Autodesk Inventor part; units mm, degrees
ref_plane "YZ Plane" through (0, 0, 0) normal (1, 0, 0) x (0, 1, 0)
ref_plane "XZ Plane" through (0, 0, 0) normal (0, 1, 0) x (-1, 0, 0)
ref_plane "XY Plane" through (0, 0, 0) normal (0, 0, 1) x (1, 0, 0)
sketch "Sketch1" plane through (0, 0, 0) normal (0, 0, 1) x (1, 0, 0)
  line L0 (-32.5, 16.5) -> (32.5, 16.5)
  line L1 (32.5, 16.5) -> (32.5, -16.5)
  line L2 (32.5, -16.5) -> (-32.5, -16.5)
  line L3 (-32.5, -16.5) -> (-32.5, 16.5)
  line L4 (-32.5, 16.5) -> (32.5, -16.5) construction
  line L5 (32.5, 16.5) -> (-32.5, -16.5) construction
  point P0 (0, 0)
  dimension "d0" = 65
  dimension "d1" = 33
extrude "Extrusion1" add sketch "Sketch1" along normal blind 66
shell "Shell1" thickness 3 removed faces 1 at (-10.8333, 5.5, 66)
sketch "Sketch2" plane through (-32.5, -16.5, 0) normal (0, -1, 0) x (1, 0, 0)
  line L0 (33.5, 65) -> (31.5, 65)
  line L1 (27.5, 61) -> (27.5, 9)
  line L2 (31.5, 5) -> (33.5, 5)
  line L3 (37.5, 9) -> (37.5, 61)
  line L4 (32.5, 0) -> (32.5, 66) construction
  line L5 (65, 66) -> (0, 66)
  line L6 (0, 0) -> (65, 0)
  arc A0 (33.5, 5) -> (37.5, 9) centre (33.5, 9) ccw
  arc A1 (27.5, 9) -> (31.5, 5) centre (31.5, 9) ccw
  arc A2 (37.5, 61) -> (33.5, 65) centre (33.5, 61) ccw
  arc A3 (31.5, 65) -> (27.5, 61) centre (31.5, 61) ccw
  point P0 (37.5, 65)
  point P1 (27.5, 65)
  point P2 (27.5, 5)
  point P3 (37.5, 5)
  dimension "d5" = 10
  dimension "d6" = 60
  dimension "d7" = 5
  dimension "d10" = 4
extrude "Extrusion2" cut sketch "Sketch2" against normal up to surface (30 mm away)
sketch "Sketch3" plane through (0, 0, 0) normal (0, 0, -1) x (-1, 0, 0)
  line L0 (32.5, 16.5) -> (32.5, -16.5)
  line L1 (32.5, 0) -> (-32.5, 0) construction
  line L2 (-32.5, -16.5) -> (-32.5, 16.5)
  circle A0 centre (-15, -8) radius 2.5
  circle A1 centre (-15, 8) radius 2.5
  circle A2 centre (15, -8) radius 2.5
  circle A3 centre (15, 8) radius 2.5
  point P0 (0, 0)
  point P1 (0, 0)
  dimension "d11" = 5
  dimension "d12" = 5
  dimension "d13" = 5
  dimension "d14" = 5
  dimension "d15" = 8
  dimension "d16" = 8
  dimension "d17" = 30
  dimension "d18" = 15
extrude "Extrusion3" cut sketch "Sketch3" against normal through all
properties part number "SLIDER" material "Steel, Alloy"
Input: part model. Units: mm. Frame: model coordinates. A direction names the side the tool comes from. Give positions to 0.01 mm unless a question says otherwise; leave off trailing zeros. Order: outer loops, then holes, each group sorted by start corner. A loop starts at its lowest first (then second) coordinate and runs counter-clockwise, first axis right, second up. Notation, with made-up numbers: (16.25, -23.5) -> (68.25, -23.5) arc R27 ccw to (68.25, -1.5) -> close; hole circle Ø1 at (-33.75, 12). An arc over 180 degrees is marked (long way). Write each question's results on one line, items separated by ' | '. Start each with the question number.
Item 1: Contact query for a flat-ended pin moving along its axis: P1, Ø8, axis at x = 5.5, y = -2, coming from the +Z side. Output: stop coordinate, or through.
Item 2: Line query: line 1 (Y direction, x = -15, z = 1); line 2 (X direction, y = 5.5, z = 53); line 3 (Y direction, x = 21.5, z = 33.5). Output: solid intervals per line, ascending.
Item 3: Set-up query: faces 4 (the flat face through (8, -16.5, 33)), 5 (the flat face through (29.5, 0, 34)), 6 (the flat face through (0, -15, 65)). Return all of +Z, -Z, +X, -X, +Y, -Y with unobstructed straight access to the full face (end or side cutting, diameter ignored); none if empty.
Item 4: Cut plane D-D on y = -1. Return the cut outline in (x, z).
Item 5: Cut plane B-B on x = 18.5. Return the cut outline in (y, z).
Item 6: Mould query, pull axis Y, two halves, no side actions, for faces 1 (the flat face through (0, 16.5, 33)), 2 (the cylindrical face through (3.797, -15.021, 6.141)), 3 (the cylindrical face through (17, -9.5, 1.5)). Classes: pulls with the +Y half, pulls with the -Y half, needs draft (parallel to the pull), parting line crosses it, or undercut.
Item 7: Cut plane A-A on y = -8. Return the cut outline in (x, z), then the cut area to 3 significant figures.
Item 8: Cut plane C-C on x = -15. Return the cut outline in (y, z), then the cut area to 3 significant figures.
Established:
1) P1: z = 3
2) line 1: -16.5 to -10.5, -5.5 to 5.5, 10.5 to 16.5 | line 2: -32.5 to -29.5, 29.5 to 32.5 | line 3: -16.5 to -13.5, 13.5 to 16.5
3) face 4: +Z, -Z, +X, -X, -Y | face 5: +Z | face 6: -Y
4) outline: (-32.5, 0) -> (32.5, 0) -> (32.5, 66) -> (29.5, 66) -> (29.5, 3) -> (-29.5, 3) -> (-29.5, 66) -> (-32.5, 66) -> close
5) outline: (-16.5, 0) -> (16.5, 0) -> (16.5, 66) -> (13.5, 66) -> (13.5, 3) -> (-13.5, 3) -> (-13.5, 66) -> (-16.5, 66) -> close
6) face 1: pulls with the +Y half | face 2: needs draft | face 3: undercut
7) outline: (-32.5, 0) -> (-17.5, 0) -> (-17.5, 3) -> (-29.5, 3) -> (-29.5, 66) -> (-32.5, 66) -> close; (-12.5, 0) -> (12.5, 0) -> (12.5, 3) -> (-12.5, 3) -> close; (17.5, 0) -> (32.5, 0) -> (32.5, 66) -> (29.5, 66) -> (29.5, 3) -> (17.5, 3) -> close | area: 543 mm^2
8) outline: (-16.5, 0) -> (-10.5, 0) -> (-10.5, 3) -> (-13.5, 3) -> (-13.5, 66) -> (-16.5, 66) -> close; (-5.5, 0) -> (5.5, 0) -> (5.5, 3) -> (-5.5, 3) -> close; (10.5, 0) -> (16.5, 0) -> (16.5, 66) -> (13.5, 66) -> (13.5, 3) -> (10.5, 3) -> close | area: 447 mm^2
